```python
from build123d import *

# Parameters (mm, degrees)
SKETCH_1_R               = 15
SKETCH_1_R_2             = 10
SKETCH_1_R_3             = 1.070370935
EXTRUDE_2_DEPTH          = 3
EXTRUDE_7_DEPTH          = 220.766502815
EXTRUDE_7_DEPTH_BACK     = 3
SKETCH_3_R               = 10
SKETCH_6_W               = 32.150004278
SKETCH_6_H               = 24.543060803
EXTRUDE_8_DEPTH          = 13
SKETCH_7_R               = 9.2
CUT_EXTRUDE_1_DEPTH      = 44
CUT_EXTRUDE_2_DEPTH      = 218
FILLET_1_R               = 1
FILLET_2_R               = 1
FILLET_3_R               = 1
EXTRUDE_9_DEPTH          = 15
EXTRUDE_9_DEPTH_BACK     = 2
SKETCH_10_W              = 8.615383554
SKETCH_10_H              = 30.150004278
CUT_EXTRUDE_3_DEPTH      = 265
CUT_EXTRUDE_4_DEPTH      = 10
CUT_EXTRUDE_4_DEPTH_BACK = 111
SKETCH_12_W              = 40.878647102
SKETCH_12_H              = 15
SKETCH_13_R              = 12
EXTRUDE_10_DEPTH         = 3
SKETCH_14_R              = 1.49
CUT_EXTRUDE_5_DEPTH      = 25


with BuildPart() as part:
    # 草图1 → 凸台-拉伸2 (new body)
    with BuildSketch(Plane(origin=(0, 0, 0), x_dir=(1, 0, 0), z_dir=(0, 1, 0))):
        with Locations(Location((0, 0, 0), (0, 0, 270))):
            Circle(SKETCH_1_R)
        with Locations(Location((0, 0, 0), (0, 0, 270))):
            Circle(SKETCH_1_R_2, mode=Mode.SUBTRACT)
        with Locations(Location((12, 0, 0), (0, 0, 270))):
            Circle(SKETCH_1_R_3, mode=Mode.SUBTRACT)
        with Locations(Location((-12, 0, 0), (0, 0, 270))):
            Circle(SKETCH_1_R_3, mode=Mode.SUBTRACT)
        with Locations(Location((0, 12, 0), (0, 0, 270))):
            Circle(SKETCH_1_R_3, mode=Mode.SUBTRACT)
        with Locations(Location((0, -12, 0), (0, 0, 270))):
            Circle(SKETCH_1_R_3, mode=Mode.SUBTRACT)
    extrude(amount=EXTRUDE_2_DEPTH)

    # 草图3 → 凸台-拉伸7 (add, two sides: drawn at the far end of the back side and taken through both)
    with BuildSketch(Plane(origin=(0, 3, 0), x_dir=(1, 0, 0), z_dir=(0, 1, 0)).offset(-EXTRUDE_7_DEPTH_BACK)):
        with Locations(Location((0, 0, 0), (0, 0, 270))):
            Circle(SKETCH_3_R)
    extrude(amount=EXTRUDE_7_DEPTH + EXTRUDE_7_DEPTH_BACK)

    # 草图6 → 凸台-拉伸8 (add)
    with BuildSketch(Plane(origin=(65.479343136, 17.545137114, 0), x_dir=(0, 0, 1), z_dir=(-0.9659258262890673, -0.25881904510252474, 0))):
        with Locations((0.609852797, 225.767598204)):
            Rectangle(SKETCH_6_W, SKETCH_6_H)
    extrude(amount=EXTRUDE_8_DEPTH)

    # 草图7 → 切除-拉伸1 (cut)
    with BuildSketch(Plane(origin=(65.479343136, 17.545137114, 0), x_dir=(0, 0, -1), z_dir=(0.9659258262890673, 0.25881904510252474, 0))):
        with Locations(Location((0, 225.99664207, 0), (0, 0, 90))):
            Circle(SKETCH_7_R)
    extrude(amount=-CUT_EXTRUDE_1_DEPTH, mode=Mode.SUBTRACT)

    # 草图8 → 切除-拉伸2 (cut)
    with BuildSketch(Plane(origin=(0, 223.766502815, 0), x_dir=(1, 0, 0), z_dir=(0, 1, 0))):
        Polygon((-8.686752569, 5.062170738), (-8.608116415, -5.089236857), (-12.71958383, -5.121085641), (-12.798219984, 5.030321955), align=None)
    extrude(amount=-CUT_EXTRUDE_2_DEPTH, mode=Mode.SUBTRACT)

    # 圆角1
    fillet_1_edges = [part.edges().sort_by_distance(p)[0] for p in [
        (-2.408234698, 245.790955307, -15.465149342),
        (3.870283173, 247.473279101, 0.609852797),
        (-2.408234698, 245.790955307, 16.684854936),
        (-8.686752569, 244.108631514, 0.609852797),
    ]]
    fillet(fillet_1_edges, radius=FILLET_1_R)

    # 圆角2
    # the kernel refuses this fillet: 1 mm, written as the material it takes off along each edge
    with BuildSketch(Plane(origin=(3.163176392, 246.248534229, -14.465149342), x_dir=(0.9659258262890673, 0.25881904510252474, 0), z_dir=(0, 0, -1))) as fillet_2_piece_1_section:
        Polygon((0, 0), (FILLET_2_R * 1.02, 0), (FILLET_2_R * 1.02, -FILLET_2_R * 1.02), (0, -FILLET_2_R * 1.02), align=None)
    fillet_2_piece_1 = extrude(amount=FILLET_2_R * 1.02, mode=Mode.PRIVATE)
    fillet_2_piece_1 = fillet_2_piece_1 - Plane(origin=(3.163176392, 246.248534229, -14.465149342), x_dir=(-0.49999999999999645, -0.8660254037844407, 0), z_dir=(0, 0, -1)) * Sphere(FILLET_2_R, mode=Mode.PRIVATE)
    add(fillet_2_piece_1, mode=Mode.SUBTRACT)
    with BuildSketch(Plane(origin=(-7.462007697, 243.401524733, -14.465149342), x_dir=(0, 0, -1), z_dir=(-0.9659258262890673, -0.25881904510252474, 0))) as fillet_2_piece_2_section:
        Polygon((0, 0), (FILLET_2_R * 1.02, 0), (FILLET_2_R * 1.02, -FILLET_2_R * 1.02), (0, -FILLET_2_R * 1.02), align=None)
    fillet_2_piece_2 = extrude(amount=FILLET_2_R * 1.02, mode=Mode.PRIVATE)
    fillet_2_piece_2 = fillet_2_piece_2 - Plane(origin=(-7.462007697, 243.401524733, -14.465149342), x_dir=(0.1830127018922222, -0.6830127018922186, 0.7071067811865475), z_dir=(-0.9659258262890673, -0.25881904510252474, 0)) * Sphere(FILLET_2_R, mode=Mode.PRIVATE)
    add(fillet_2_piece_2, mode=Mode.SUBTRACT)
    with BuildSketch(Plane(origin=(-7.462007697, 243.401524733, 15.684854936), x_dir=(0, 0, 1), z_dir=(-0.9659258262890673, -0.25881904510252474, 0))) as fillet_2_piece_3_section:
        Polygon((0, 0), (FILLET_2_R * 1.02, 0), (FILLET_2_R * 1.02, FILLET_2_R * 1.02), (0, FILLET_2_R * 1.02), align=None)
    fillet_2_piece_3 = extrude(amount=FILLET_2_R * 1.02, mode=Mode.PRIVATE)
    fillet_2_piece_3 = fillet_2_piece_3 - Plane(origin=(-7.462007697, 243.401524733, 15.684854936), x_dir=(0.18301270189222205, -0.6830127018922186, -0.7071067811865475), z_dir=(-0.9659258262890673, -0.25881904510252474, 0)) * Sphere(FILLET_2_R, mode=Mode.PRIVATE)
    add(fillet_2_piece_3, mode=Mode.SUBTRACT)
    with BuildSketch(Plane(origin=(3.163176392, 246.248534229, 15.684854936), x_dir=(0.9659258262890673, 0.25881904510252474, 0), z_dir=(0, 0, 1))) as fillet_2_piece_4_section:
        Polygon((0, 0), (FILLET_2_R * 1.02, 0), (FILLET_2_R * 1.02, FILLET_2_R * 1.02), (0, FILLET_2_R * 1.02), align=None)
    fillet_2_piece_4 = extrude(amount=FILLET_2_R * 1.02, mode=Mode.PRIVATE)
    fillet_2_piece_4 = fillet_2_piece_4 - Plane(origin=(3.163176392, 246.248534229, 15.684854936), x_dir=(-0.49999999999999645, -0.8660254037844407, 0), z_dir=(0, 0, 1)) * Sphere(FILLET_2_R, mode=Mode.PRIVATE)
    add(fillet_2_piece_4, mode=Mode.SUBTRACT)
    with BuildSketch(Plane(origin=(-1.627434227, 221.6266001, 15.684854936), x_dir=(0, 0, 1), z_dir=(-0.9659258262890673, -0.25881904510252474, 0))) as fillet_2_piece_5_section:
        Polygon((0, 0), (FILLET_2_R * 1.02, 0), (FILLET_2_R * 1.02, -FILLET_2_R * 1.02), (0, -FILLET_2_R * 1.02), align=None)
    fillet_2_piece_5 = extrude(amount=FILLET_2_R * 1.02, mode=Mode.PRIVATE)
    fillet_2_piece_5 = fillet_2_piece_5 - Plane(origin=(-1.627434227, 221.6266001, 15.684854936), x_dir=(-0.1830127018922222, 0.6830127018922186, -0.7071067811865475), z_dir=(-0.9659258262890673, -0.25881904510252474, 0)) * Sphere(FILLET_2_R, mode=Mode.PRIVATE)
    add(fillet_2_piece_5, mode=Mode.SUBTRACT)
    with BuildSketch(Plane(origin=(12.6373093, 224.413550428, -15.465149342), x_dir=(0, 0, 1), z_dir=(-0.9659258262890673, -0.25881904510252474, 0))) as fillet_2_piece_6:
        with BuildLine():
            CenterArc((FILLET_2_R, FILLET_2_R), FILLET_2_R, 180, 90)
            Line((0, FILLET_2_R), (0, 0))
            Line((0, 0), (FILLET_2_R, 0))
        make_face()
    extrude(amount=18, mode=Mode.SUBTRACT)
    with BuildSketch(Plane(origin=(4.129102218, 246.507353274, -15.465149342), x_dir=(-0.9659258262890672, -0.2588190451025247, 0), z_dir=(0.25881904510252474, -0.9659258262890673, 0)), Plane(origin=(-8.427933524, 243.142705688, -15.465149342), x_dir=(0, 0, 1), z_dir=(0.25881904510252474, -0.9659258262890673, 0)), Plane(origin=(10.869542347, 221.35168825, 16.684854936), x_dir=(-0.9659258262890672, -0.2588190451025247, 0), z_dir=(-0.25881904510252474, 0.9659258262890673, 0))) as fillet_2_piece_7:
        with BuildLine():
            CenterArc((FILLET_2_R, -FILLET_2_R), FILLET_2_R, 90, 90)
            Line((0, -FILLET_2_R), (0, 0))
            Line((0, 0), (FILLET_2_R, 0))
        make_face()
    extrude(amount=26.043060803, mode=Mode.SUBTRACT)
    with BuildSketch(Plane(origin=(12.6373093, 224.413550428, 16.684854936), x_dir=(-0.2588190451025247, 0.9659258262890672, 0), z_dir=(-0.9659258262890673, -0.25881904510252474, 0))) as fillet_2_piece_8:
        with BuildLine():
            CenterArc((FILLET_2_R, FILLET_2_R), FILLET_2_R, 180, 90)
            Line((0, FILLET_2_R), (0, 0))
            Line((0, 0), (FILLET_2_R, 0))
        make_face()
    extrude(amount=14.5, mode=Mode.SUBTRACT)
    with BuildSketch(Plane(origin=(-2.593360053, 221.367781055, 16.684854936), x_dir=(0, 0, -1), z_dir=(-0.25881904510252474, 0.9659258262890673, 0))) as fillet_2_piece_9:
        with BuildLine():
            CenterArc((FILLET_2_R, -FILLET_2_R), FILLET_2_R, 90, 90)
            Line((0, -FILLET_2_R), (0, 0))
            Line((0, 0), (FILLET_2_R, 0))
        make_face()
    extrude(amount=22.543060803, mode=Mode.SUBTRACT)
    with BuildSketch(Plane(origin=(-2.334541008, 220.401855229, 7.223678228), x_dir=(-0.2588190451025276, 0.9659258262890665, 0), z_dir=(0, 0, 1))) as fillet_2_piece_10_section:
        with BuildLine():
            CenterArc((FILLET_2_R, -FILLET_2_R), FILLET_2_R, 90, 90)
            Line((0, -FILLET_2_R), (0, 0))
            Line((0, 0), (FILLET_2_R, 0))
        make_face()
    fillet_2_piece_10 = extrude(amount=8.461176708, mode=Mode.PRIVATE)
    fillet_2_piece_10 = fillet_2_piece_10 - Plane(origin=(0, 220.67611038, 0), x_dir=(0, 0, 1), z_dir=(0, -1, 0)) * Cylinder(10, 21, mode=Mode.PRIVATE)
    add(fillet_2_piece_10, mode=Mode.SUBTRACT)

    # 圆角3
    # the kernel refuses this fillet: 1 mm, written as the material it takes off along each edge
    with BuildSketch(Plane(origin=(-1.627434227, 221.6266001, -14.465149342), x_dir=(0.25881904510252474, -0.9659258262890673, 0), z_dir=(-0.9659258262890673, -0.25881904510252474, 0))) as fillet_3_piece_1_section:
        Polygon((0, 0), (FILLET_3_R, 0), (FILLET_3_R, -FILLET_3_R), (0, -FILLET_3_R), align=None)
    fillet_3_piece_1 = extrude(amount=FILLET_3_R, mode=Mode.PRIVATE)
    fillet_3_piece_1 = fillet_3_piece_1 - Plane(origin=(-1.627434227, 221.6266001, -14.465149342), x_dir=(-0.18301270189222205, 0.6830127018922186, 0.7071067811865475), z_dir=(-0.9659258262890673, -0.25881904510252474, 0)) * Sphere(FILLET_3_R, mode=Mode.PRIVATE)
    add(fillet_3_piece_1, mode=Mode.SUBTRACT)
    with BuildSketch(Plane(origin=(-2.334541008, 220.401855229, -14.465149342), x_dir=(-0.2588190451025293, 0.9659258262890661, 0), z_dir=(0, 0, 1))) as fillet_3_piece_2_section:
        with BuildLine():
            CenterArc((FILLET_3_R, -FILLET_3_R), FILLET_3_R, 90, 90)
            Line((0, -FILLET_3_R), (0, 0))
            Line((0, 0), (FILLET_3_R, 0))
        make_face()
    fillet_3_piece_2 = extrude(amount=7.241471114, mode=Mode.PRIVATE)
    fillet_3_piece_2 = fillet_3_piece_2 - Plane(origin=(0, 220.680283856, 0), x_dir=(0, 0, 1), z_dir=(0, -1, 0)) * Cylinder(10, 19, mode=Mode.PRIVATE)
    add(fillet_3_piece_2, mode=Mode.SUBTRACT)

    # 草图9 → 凸台-拉伸9 (add, two sides: drawn at the far end of the back side and taken through both)
    with BuildSketch(Plane(origin=(65.479343136, 17.545137114, 0), x_dir=(0, 0, 1), z_dir=(-0.9659258262890673, -0.25881904510252474, 0)).offset(-EXTRUDE_9_DEPTH_BACK)):
        Polygon((-15.465149342, 214.521357737), (-4.839983079, 214.521357737), (-4.955271508, 194.209196023), align=None)
        Polygon((16.619377138, 214.521357737), (5.079909852, 214.521357737), (5.089236857, 193.804302434), align=None)
    extrude(amount=EXTRUDE_9_DEPTH + EXTRUDE_9_DEPTH_BACK)

    # 草图10 → 切除-拉伸3 (cut)
    with BuildSketch(Plane(origin=(0, 3, 0), x_dir=(1, 0, 0), z_dir=(0, 1, 0))):
        with Locations((14.264821949, -0.609852797)):
            Rectangle(SKETCH_10_W, SKETCH_10_H)
    extrude(amount=CUT_EXTRUDE_3_DEPTH, mode=Mode.SUBTRACT)

    # 草图12 → 切除-拉伸4 (cut, two sides: drawn at the far end of the back side and taken through both)
    with BuildSketch(Plane(origin=(-8.647020453, 0, 0.066982674), x_dir=(0.007746097662068172, 0, 0.999969998535461), z_dir=(-0.999969998535461, 0, 0.007746097662068172)).offset(-CUT_EXTRUDE_4_DEPTH_BACK)):
        with Locations((1.109642623, 7.5)):
            Rectangle(SKETCH_12_W, SKETCH_12_H)
    extrude(amount=CUT_EXTRUDE_4_DEPTH + CUT_EXTRUDE_4_DEPTH_BACK, mode=Mode.SUBTRACT)

    # 草图13 → 凸台-拉伸10 (add)
    with BuildSketch(Plane.XZ.offset(-15)):
        with Locations(Location((0, 0, 0), (0, 0, 270))):
            Circle(SKETCH_13_R)
    extrude(amount=-EXTRUDE_10_DEPTH)

    # 草图14 → 切除-拉伸5 (cut)
    with BuildSketch(Plane(origin=(0, 15, 0), x_dir=(-1, 0, 0), z_dir=(0, -1, 0))):
        with Locations(Location((0, 0, 0), (0, 0, 90))):
            Circle(SKETCH_14_R)
    extrude(amount=-CUT_EXTRUDE_5_DEPTH, mode=Mode.SUBTRACT)


solid = part.part
```
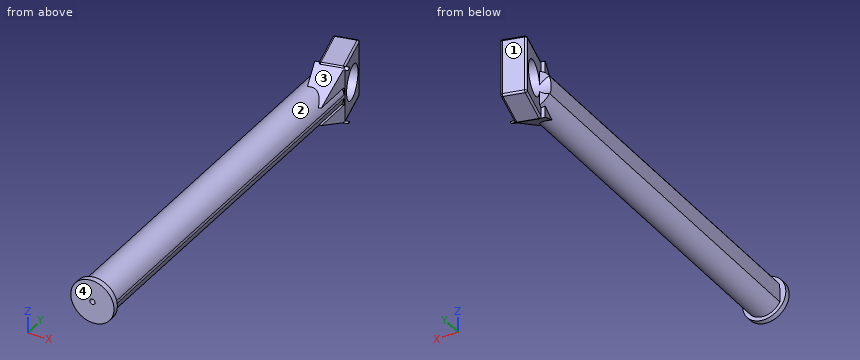
Geometry: final body of the model. Coordinates: model frame, mm. Face numbers are marked on the shaded views. Round coordinates to 2 decimals unless told otherwise and drop trailing zeros. Order: outer loops, then holes, each group sorted by start corner. A loop starts at its lowest first (then second) coordinate and runs counter-clockwise, first axis right, second up. Notation, with made-up numbers: M 60,58.5 L 96,58.5 A14 cw 96,82.5 Z; hole C 17,-24 d10. An arc over 180 degrees is marked long. One line per item, written item: value.
(1) Pull-direction query (Y, two-part tool) for the marked faces 1, 2, 3 and 4; classes: pulls with the +Y half, pulls with the -Y half, needs draft (parallel to the pull), parting line crosses it, or undercut.
Result sheet:
face 1: pulls with the +Y half
face 2: undercut
face 3: undercut
face 4: pulls with the -Y half
(2) Line query: probe 1 along X at (y, z) = (24, 0); probe 2 along Y at (x, z) = (10.75, -3.5); probe 3 along X at (y, z) = (176, 5). Output: solid intervals per line, ascending. Write a range as [from, to].
Result sheet:
probe 1: [-8.65, -1.49], [1.49, 9.96]
probe 2: [15, 18]
probe 3: [-8.61, 8.66]
(3) Cut plane A-A (y = 97.5). Return the cut outline in (x, z), and give its area (3 significant figures).
Result sheet:
outline: M -8.69,-4.96 A10 ccw 9.96,-0.92 L 9.96,0.92 A10 ccw -8.61,5.09 Z
area: 305 mm2
(4) Pin query (flat end, axial travel): P1, Ø8, axis at x = -1.5, z = -3.5, coming from the +Y side; P2, Ø6, axis at x = -5.5, z = -4.5, coming from the +Y side; P3, Ø2.5, axis at x = 0, z = 0, coming from the +Y side. Return the tip coordinate at first contact, or that it passes through.
Result sheet:
P1: y = 247.11
P2: y = 245.77
P3: y = 246.77
